```python
from build123d import *

# Parameters (mm, degrees)
SKETCH3_R                 = 44
BOSS_EXTRUDE1_DEPTH       = 1.25
SKETCH4_W                 = 100.44
SKETCH4_H                 = 1.25
BOSS_EXTRUDE2_DEPTH       = 2
BOSS_EXTRUDE3_OUTLINE_R   = 4.5
BOSS_EXTRUDE3_OUTLINE_R_2 = 2.25
BOSS_EXTRUDE3_DEPTH       = 28.5


with BuildPart() as part:
    # Sketch1 → Loft1 section 0
    with BuildSketch(Plane(origin=(0, 0, 0), x_dir=(1, 0, 0), z_dir=(0, 1, 0))):
        with BuildLine():
            Line((47.68, 0), (47.68, -47))
            ThreePointArc((47.68, -47), (0, -94.68), (-47.68, -47))
            Line((-47.68, -47), (-47.68, 0))
            Line((-47.68, 0), (-50.22, 0))
            Line((-50.22, 0), (-50.22, -47))
            ThreePointArc((-50.22, -47), (0, -97.22), (50.22, -47))
            Line((50.22, -47), (50.22, 0))
            Line((50.22, 0), (47.68, 0))
        make_face()
    # Sketch2 → Loft1 section 1
    with BuildSketch(Plane(origin=(0, 34, 0), x_dir=(1, 0, 0), z_dir=(0, 1, 0))):
        with BuildLine():
            Line((-56.04, 0), (-56.04, -46.2))
            ThreePointArc((-56.04, -46.2), (0, -102.24), (56.04, -46.2))
            Line((56.04, -46.2), (56.04, 0))
            Line((56.04, 0), (53.5, 0))
            Line((53.5, 0), (53.5, -46.2))
            ThreePointArc((53.5, -46.2), (0, -99.7), (-53.5, -46.2))
            Line((-53.5, -46.2), (-53.5, 0))
            Line((-53.5, 0), (-56.04, 0))
        make_face()
    loft()

    # Sketch3 → Boss-Extrude1 (add)
    with BuildSketch(Plane.XZ):
        with BuildLine():
            Line((-50.219775987, 0), (50.219775987, 0))
            Line((50.219775987, 0), (50.219775987, 46.850000669))
            ThreePointArc((50.219775987, 46.850000669), (0, 96.920001338), (-50.219775987, 46.850000669))
            Line((-50.219775987, 46.850000669), (-50.219775987, 0))
        make_face()
        with Locations(Location((0, 47, 0), (0, 0, 270))):
            Circle(SKETCH3_R, mode=Mode.SUBTRACT)
    extrude(amount=-BOSS_EXTRUDE1_DEPTH)

    # Sketch4 → Boss-Extrude2 (add)
    with BuildSketch(Plane(origin=(0, 1.25, 0), x_dir=(1, 0, 0), z_dir=(0, 1, 0))):
        with Locations((0, -0.625)):
            Rectangle(SKETCH4_W, SKETCH4_H)
    extrude(amount=BOSS_EXTRUDE2_DEPTH)

    # Boss-Extrude3: read off the stored shape, not the designer's step
    # Boss-Extrude3 outline → Boss-Extrude3 (add)
    with BuildSketch(Plane(origin=(0, 1.25, 0), x_dir=(1, 0, 0), z_dir=(0, 1, 0))):
        with Locations((-42.713936364, -23)):
            Circle(BOSS_EXTRUDE3_OUTLINE_R)
        with Locations((-42.713936364, -23)):
            Circle(BOSS_EXTRUDE3_OUTLINE_R_2, mode=Mode.SUBTRACT)
    boss_extrude3 = extrude(amount=BOSS_EXTRUDE3_DEPTH)

    # Mirror1: Boss-Extrude3 across plane
    add(boss_extrude3.mirror(Plane(origin=(0, 0, 0), x_dir=(0, 0, 1), z_dir=(1, 0, 0))))


solid = part.part
```
Model file for the job. Use its own axes, mm. A direction names the side the tool comes from. Round coordinates to 2 decimals unless told otherwise and drop trailing zeros. Use CSV: the item, a comma, the result in double quotes. Start each with the question number.
Item 1: Two-plate mould, pull along X, no slides. Class faces 4 (the face through (-4, 0, 2)), 5 (the face through (-40.636, 15.3, 23.862)): released by +X, released by -X, zero draft, split by the parting line, or undercut.
Item 2: Tool access for faces 1 (the face through (7, 3, 0)), 2 (the face through (7, 1.25, 3)), 3 (the face through (-45, 29.75, 24)): list every direction of +Z, -Z, +X, -X, +Y, -Y with a clear straight run to the whole face (end or side of a thin tool).
Item 3: Band-saw the part on A-A (y = 27.5). State how many separate pieces and enclosed holes the cut face has, and give its area (3 significant figures).
Item 4: Pin check, flat tips, straight feed: P1, Ø1, axis at x = 16.5, z = 1, coming from the +Y side; P2, Ø5, axis at x = 42.71, z = 23, coming from the +Y side; P3, Ø2, axis at x = -18, y = 2.5, coming from the +Z side. Stop position of each tip, or through.
Item 5: Drill centre lines: L1, parallel to X at y = 12, z = 23; L2, parallel to X at y = 20.5, z = 90; L3, parallel to Z at x = 42, y = 29. Where is each one in solid material? Low to high. Write a range as [from, to].
Checked values:
1,face 4,"zero draft"
1,face 5,"undercut"
2,face 1,"-Z, +X, -X, +Y, -Y"
2,face 2,"+Y"
2,face 3,"-Z, +Y"
3,separate pieces,"3"
3,enclosed holes,"2"
3,area,"759 mm²"
4,P1,"stops at y = 3.25"
4,P2,"stops at y = 29.75"
4,P3,"stops at z = 94.68"
5,L1,"x = [-52.27, -49.73], [-47.21, -44.96], [-40.46, -38.21], [38.21, 40.46], [44.96, 47.21], [49.73, 52.27]"
5,L2,"x = [-31.56, -27.01], [27.01, 31.56]"
5,L3,"z = [18.56, 20.87], [25.13, 27.44], [78.06, 82.11]"
